Check sheet for the modelled part. Datum: model origin and axes. Units: mm. Face numbers are marked on the shaded views. A direction names the side the tool comes from. Give positions to 0.01 mm unless a question says otherwise; leave off trailing zeros. Write each loop counter-clockwise with the first axis right and the second up, starting at its lowest first coordinate (ties: lowest second). Pieces come first, ordered by that corner, then holes. Notation, with made-up numbers: (14.5, 82.25) -> (71.5, 82.25) arc R22 cw to (71.5, 100.25) -> close; hole circle Ø11 at (57.25, 52). An arc over 180 degrees is marked (long way). Answer as a JSON object with one key per item and string values.
from build123d import *

# Parameters (mm, degrees)
F0_R     = 5
F1_DEPTH = 100
F2_R     = 7.5
F3_DEPTH = 10
F4_SIZE  = 0.5


with BuildPart() as f1:
    # F0 (on Right) → F1 (new body)
    with BuildSketch(Plane.YZ):
        Circle(F0_R)
    extrude(amount=-F1_DEPTH)

    # F2 (on Right) → F3 (join)
    with BuildSketch(Plane.YZ):
        Circle(F2_R)
    extrude(amount=F3_DEPTH)

    # F4
    f4_edges = [f1.edges().sort_by_distance(p)[0] for p in [
        (10, -7.5, 0),
        (-100, -5, 0),
        (0, -7.5, 0),
    ]]
    chamfer(f4_edges, length=F4_SIZE)


solid = f1.part
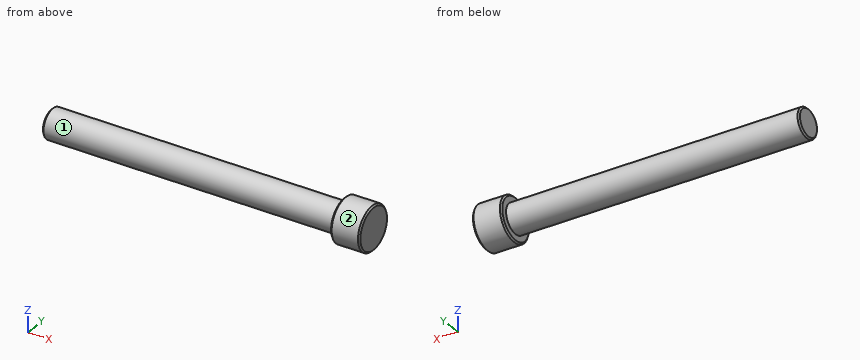
1. Sectioned sample at A-A, the plane y = 0. Enter the section's corners in (x, z).
Determined:
{"outline": "(-100, -4.5) -> (-99.5, -5) -> (0, -5) -> (0, -7) -> (0.5, -7.5) -> (9.5, -7.5) -> (10, -7) -> (10, 7) -> (9.5, 7.5) -> (0.5, 7.5) -> (0, 7) -> (0, 5) -> (-99.5, 5) -> (-100, 4.5) -> close"}
2. Scan lines: L1, parallel to X at y = 3.5, z = -4.5; L2, parallel to X at y = -3, z = -6.75; L3, parallel to Z at x = 2, y = 6. Record each from-to range of solid material in increasing order. Write a range as [from, to].
Determined:
{"L1": "[0, 10]", "L2": "[0.39, 9.61]", "L3": "[-4.5, 4.5]"}
3. Go/stop test with flat-tipped pins: P1, Ø5, axis at x = -46.5, z = 3, coming from the +Y side; P2, Ø1, axis at y = -5, z = 1, coming from the -X side; P3, Ø4, axis at x = -76, z = 2.5, coming from the -Y side. Record where each tip stops, or that it passes through.
Determined:
{"P1": "y = 4.97", "P2": "x = -99.9", "P3": "y = -4.97"}
4. Sectioned sample at C-C, the plane x = -74.5. Enter the section's corners in (y, z).
Determined:
{"outline": "circle Ø10 at (0, 0)"}
5. Access from +Z, -Z, +X, -X, +Y, -Y to the whole of each face (thin tool, end or side, straight path). Record for the marked faces 1 and 2.
Determined:
{"face 1": "-X", "face 2": "+X, -X"}
